```python
from build123d import *

# Parameters (mm, degrees)
SKETCH2_W               = 76.2
SKETCH2_H               = 50.8
BOSS_EXTRUDE2_DEPTH     = 3.175
CUT_EXTRUDE1_DEPTH      = 47.228697797
CUT_EXTRUDE1_DEPTH_BACK = 47.228697797
CUT_EXTRUDE3_START      = -3.175
CUT_EXTRUDE3_DEPTH      = 3.175
CUT_EXTRUDE2_DEPTH      = 64.579325453
CUT_EXTRUDE2_DEPTH_BACK = 15.24
SKETCH4_R               = 1.27


with BuildPart() as part:
    # Sketch2 → Boss-Extrude2 (new, symmetric)
    with BuildSketch(Plane(origin=(0, 0, 0), x_dir=(0, 0, -1), z_dir=(1, 0, 0))):
        Rectangle(SKETCH2_W, SKETCH2_H)
    extrude(amount=BOSS_EXTRUDE2_DEPTH, both=True)

    # Sketch3 → Cut-Extrude1 (cut, two sides: drawn at the far end of the back side and taken through both)
    with BuildSketch(Plane(origin=(3.175, 0, 0), x_dir=(0, 0, -1), z_dir=(1, 0, 0)).offset(-CUT_EXTRUDE1_DEPTH_BACK)):
        with BuildLine():
            Line((-12.499999952, -9.525), (-12.499999952, 15.875))
            ThreePointArc((-12.499999952, 15.875), (-14, 17.375000048), (-15.500000048, 15.875))
            Line((-15.500000048, 15.875), (-15.500000048, -9.525))
            ThreePointArc((-15.500000048, -9.525), (-14, -11.025000048), (-12.499999952, -9.525))
        make_face()
        with BuildLine():
            Line((15.500000048, -9.525), (15.500000048, 15.875))
            ThreePointArc((15.500000048, 15.875), (14, 17.375000048), (12.499999952, 15.875))
            Line((12.499999952, 15.875), (12.499999952, -9.525))
            ThreePointArc((12.499999952, -9.525), (14, -11.025000048), (15.500000048, -9.525))
        make_face()
    extrude(amount=CUT_EXTRUDE1_DEPTH + CUT_EXTRUDE1_DEPTH_BACK, mode=Mode.SUBTRACT)

    # Sketch3_3 → Cut-Extrude3 (cut)
    # profile 1 of 2: a face of its own
    with BuildSketch(Plane(origin=(3.175, 0, 0), x_dir=(0, 0, -1), z_dir=(1, 0, 0)).offset(CUT_EXTRUDE3_START)):
        with BuildLine():
            Line((-18.250000009, -9.525), (-18.250000009, 15.875))
            ThreePointArc((-18.250000009, 15.875), (-14, 20.125000009), (-9.749999991, 15.875))
            Line((-9.749999991, 15.875), (-9.749999991, -9.525))
            ThreePointArc((-9.749999991, -9.525), (-14, -13.775000009), (-18.250000009, -9.525))
        make_face()
        with BuildLine():
            Line((-15.500000048, -9.525), (-15.500000048, 15.875))
            ThreePointArc((-15.500000048, 15.875), (-14, 17.375000048), (-12.499999952, 15.875))
            Line((-12.499999952, 15.875), (-12.499999952, -9.525))
            ThreePointArc((-12.499999952, -9.525), (-14, -11.025000048), (-15.500000048, -9.525))
        make_face(mode=Mode.SUBTRACT)
    # profile 2 of 2: a face of its own
    with BuildSketch(Plane(origin=(3.175, 0, 0), x_dir=(0, 0, -1), z_dir=(1, 0, 0)).offset(CUT_EXTRUDE3_START)):
        with BuildLine():
            Line((9.749999991, -9.525), (9.749999991, 15.875))
            ThreePointArc((9.749999991, 15.875), (14, 20.125000009), (18.250000009, 15.875))
            Line((18.250000009, 15.875), (18.250000009, -9.525))
            ThreePointArc((18.250000009, -9.525), (14, -13.775000009), (9.749999991, -9.525))
        make_face()
        with BuildLine():
            Line((12.499999952, -9.525), (12.499999952, 15.875))
            ThreePointArc((12.499999952, 15.875), (14, 17.375000048), (15.500000048, 15.875))
            Line((15.500000048, 15.875), (15.500000048, -9.525))
            ThreePointArc((15.500000048, -9.525), (14, -11.025000048), (12.499999952, -9.525))
        make_face(mode=Mode.SUBTRACT)
    extrude(amount=CUT_EXTRUDE3_DEPTH, mode=Mode.SUBTRACT)

    # Sketch4 → Cut-Extrude2 (cut, two sides: drawn at the far end of the back side and taken through both)
    with BuildSketch(Plane.XZ.offset(25.4).offset(-CUT_EXTRUDE2_DEPTH_BACK)):
        with Locations(Location((0, 25.4, 0), (0, 0, 90))):
            Circle(SKETCH4_R)
        with Locations(Location((0, 0, 0), (0, 0, 90))):
            Circle(SKETCH4_R)
        with Locations(Location((0, -25.4, 0), (0, 0, 90))):
            Circle(SKETCH4_R)
    extrude(amount=CUT_EXTRUDE2_DEPTH + CUT_EXTRUDE2_DEPTH_BACK, mode=Mode.SUBTRACT)


solid = part.part
```
Model file for the job. Use its own axes, mm. A direction names the side the tool comes from. Coordinates: 2 decimals unless noted, no trailing zeros. Order: outer loops, then holes, each group sorted by start corner. A loop starts at its lowest first (then second) coordinate and runs counter-clockwise, first axis right, second up. Notation, with made-up numbers: (83.5, 55.25) -> (123.5, 55.25) arc R22 ccw to (123.5, 73.25) -> close; hole circle Ø2 at (-40, 80). An arc over 180 degrees is marked (long way). Return JSON: item names as keys, results as strings.
Item 1: Mould opens along Y. For faces 6 (the face through (-1.61, -11.025, 14.033)), 7 (the face through (0, 0, -38.1)), 8 (the face through (-1.4, -25.4, 0.5)) say: pulls with the +Y half, pulls with the -Y half, needs draft (parallel to the pull), parting line crosses it, or undercut.
Model answer:
{"face 6": "undercut", "face 7": "needs draft", "face 8": "pulls with the -Y half"}
Item 2: Slice it at B-B (y = 10). Write the cut outline in (x, z) (3 decimals).
Model answer:
{"outline": "(-3.175, -38.1) -> (3.175, -38.1) -> (3.175, -18.25) -> (0, -18.25) -> (0, -15.5) -> (-3.175, -15.5) -> close; (-3.175, -12.5) -> (0, -12.5) -> (0, -9.75) -> (3.175, -9.75) -> (3.175, 9.75) -> (0, 9.75) -> (0, 12.5) -> (-3.175, 12.5) -> close; (-3.175, 15.5) -> (0, 15.5) -> (0, 18.25) -> (3.175, 18.25) -> (3.175, 38.1) -> (-3.175, 38.1) -> close"}
Item 3: Slice it at A-A (z = 14). Write the cut outline in (x, y) (3 decimals).
Model answer:
{"outline": "(-3.175, -25.4) -> (3.175, -25.4) -> (3.175, -13.775) -> (0, -13.775) -> (0, -11.025) -> (-3.175, -11.025) -> close; (-3.175, 17.375) -> (0, 17.375) -> (0, 20.125) -> (3.175, 20.125) -> (3.175, 25.4) -> (-3.175, 25.4) -> close"}
Item 4: Pin check, flat tips, straight feed: P1, Ø2.5, axis at y = 11.5, z = 15, coming from the +X side; P2, Ø2, axis at x = 0, z = 0, coming from the -Y side; P3, Ø2, axis at x = -0.5, z = 25.5, coming from the -Y side. Stop position of each tip, or through.
Model answer:
{"P1": "stops at x = 0", "P2": "stops at y = -10.16", "P3": "stops at y = -25.4"}
Item 5: 3-axis set-ups, long thin cutter, end or side, ignore diameter. For faces 1 (the face through (-0.38, -17.67, -24.19)), 2 (the face through (2, 3, -18.25)), 3 (the face through (-3.175, 0, 1)), 4 (the face through (0, 25.4, 1)), 5 (the face through (-1.61, 17.375, -14.033)): which of +Z, -Z, +X, -X, +Y, -Y reach the whole face in a straight line?
Model answer:
{"face 1": "-Y", "face 2": "+X", "face 3": "+Z, -Z, -X, +Y, -Y", "face 4": "+Z, -Z, +X, -X, +Y", "face 5": "+X, -X"}
Item 6: Slice it at C-C (y = -16). Write the cut outline in (x, z) (3 decimals), then the cut area to 3 significant figures.
Model answer:
{"outline": "(-3.175, -38.1) -> (3.175, -38.1) -> (3.175, 38.1) -> (-3.175, 38.1) -> close; hole circle Ø2.54 at (0, -25.4); hole circle Ø2.54 at (0, 0); hole circle Ø2.54 at (0, 25.4)", "area": "469 mm²"}
Item 7: Wall check: line 1 along Z through (x, y) = (2.25, 5); line 2 along Z through (x, y) = (-1.5, 12.5); line 3 along X through (y, z) = (-20.5, 25.4) (3 decimals). Give the ranges that are in metal, low to high. Write a range as from..to.
Model answer:
{"line 1": "z = -38.1..-18.25, -9.75..9.75, 18.25..38.1", "line 2": "z = -38.1..-15.5, -12.5..12.5, 15.5..38.1", "line 3": "x = -3.175..-1.27, 1.27..3.175"}
Item 8: Slice it at D-D (z = 25.4). Write the cut outline in (x, y) (3 decimals).
Model answer:
{"outline": "(-3.175, -25.4) -> (-1.27, -25.4) -> (-1.27, -10.16) -> (1.27, -10.16) -> (1.27, -25.4) -> (3.175, -25.4) -> (3.175, 25.4) -> (-3.175, 25.4) -> close"}
